Model file for the job. Use its own axes, mm. Face numbers are marked on the shaded views. A direction names the side the tool comes from. Coordinates: 2 decimals unless noted, no trailing zeros. Write each loop counter-clockwise with the first axis right and the second up, starting at its lowest first coordinate (ties: lowest second). Pieces come first, ordered by that corner, then holes.
Q1. Band-saw the part on C-C, the plane x = -33. Write the cut outline in (y, z).
Q2. Band-saw the part on A-A, the plane z = 9. Write the cut outline in (x, y), plus the area to 3 significant figures.
Q3. Drill centre lines: probe 1 along Y at (x, z) = (-34, 8.25); probe 2 along X at (y, z) = (-4, 3); probe 3 along Y at (x, z) = (-37.25, 4.75). Where is each one in solid material? Low to high.
Q4. Which spindle directions (+Z, -Z, +X, -X, +Y, -Y) get a long thin tool onto all of the face, cutting with end or side? Do the marked faces 4, 5 and 6. Say none if no direction does.
Q5. Pull direction X, two halves, no side cores. Call the marked faces 1, 2 and 3: released by +X, released by -X, zero draft, split by the parting line, or undercut.
Q6. Pin check, flat tips, straight feed: P1, Ø5, axis at y = 3, z = 8.5, coming from the +X side; P2, Ø2.5, axis at x = -33.96, y = 5.9, coming from the -Z side; P3, Ø1.5, axis at x = -39, z = 5.5, coming from the +Y side; P4, Ø1, axis at y = 0.5, z = 11.5, coming from the -X side. Stop position of each tip, or through.
Q7. Band-saw the part on B-B, the plane y = 7. Write the cut outline in (x, z) (3 decimals).
Q8. Band-saw the part on D-D, the plane y = -2. Write the cut outline in (x, z), plus the area to 3 significant figures.
from build123d import *

# Parameters (mm, degrees)
F0_R     = 1.65
F1_DEPTH = 14


with BuildPart() as f1:
    # F0 (on Top) → F1 (new body)
    with BuildSketch(Plane.XY):
        with BuildLine():
            Line((-36.955225, -4.099561), (-39.955225, -4.099561))
            Line((-39.955225, -4.099561), (-39.955225, -14.099561))
            Line((-39.955225, -14.099561), (-27.955225, -14.099561))
            Line((-27.955225, -14.099561), (-27.955225, -4.099561))
            Line((-27.955225, -4.099561), (-30.955225, -4.099561))
            Line((-30.955225, -4.099561), (-30.955225, 5.900439))
            ThreePointArc((-30.955225, 5.900439), (-33.955225, 8.900439), (-36.955225, 5.900439))
            Line((-36.955225, 5.900439), (-36.955225, -4.099561))
        make_face()
        with Locations((-33.955225, 5.900439)):
            Circle(F0_R, mode=Mode.SUBTRACT)
    extrude(amount=F1_DEPTH)


solid = f1.part
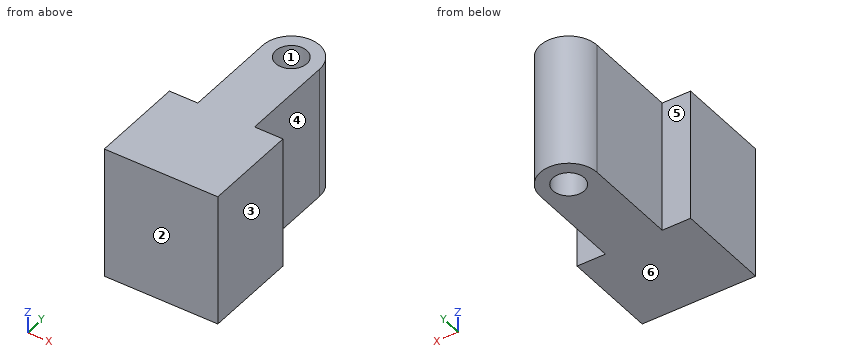
Answer sheet:
1. outline: (-14.1, 0) - (4.56, 0) - (4.56, 14) - (-14.1, 14) - close; (7.25, 0) - (8.74, 0) - (8.74, 14) - (7.25, 14) - close
2. outline: (-39.96, -14.1) - (-27.96, -14.1) - (-27.96, -4.1) - (-30.96, -4.1) - (-30.96, 5.9) arc R3 ccw to (-36.96, 5.9) - (-36.96, -4.1) - (-39.96, -4.1) - close; hole circle Ø3.3 at (-33.96, 5.9)
2. area: 186 mm2
3. probe 1: y = -14.1 to 4.25, 7.55 to 8.9
3. probe 2: x = -36.96 to -30.96
3. probe 3: y = -14.1 to -4.1
4. face 4: +Z, -Z, +X, +Y
4. face 5: +Z, -Z, -X, +Y
4. face 6: -Z, +X, -X, +Y, -Y
5. face 1: undercut
5. face 2: zero draft
5. face 3: released by +X
6. P1: stops at x = -30.96
6. P2: passes through
6. P3: stops at y = -4.1
6. P4: stops at x = -36.96
7. outline: (-36.746, 0) - (-35.185, 0) - (-35.185, 14) - (-36.746, 14) - close; (-32.725, 0) - (-31.164, 0) - (-31.164, 14) - (-32.725, 14) - close
8. outline: (-36.96, 0) - (-30.96, 0) - (-30.96, 14) - (-36.96, 14) - close
8. area: 84.0 mm2
